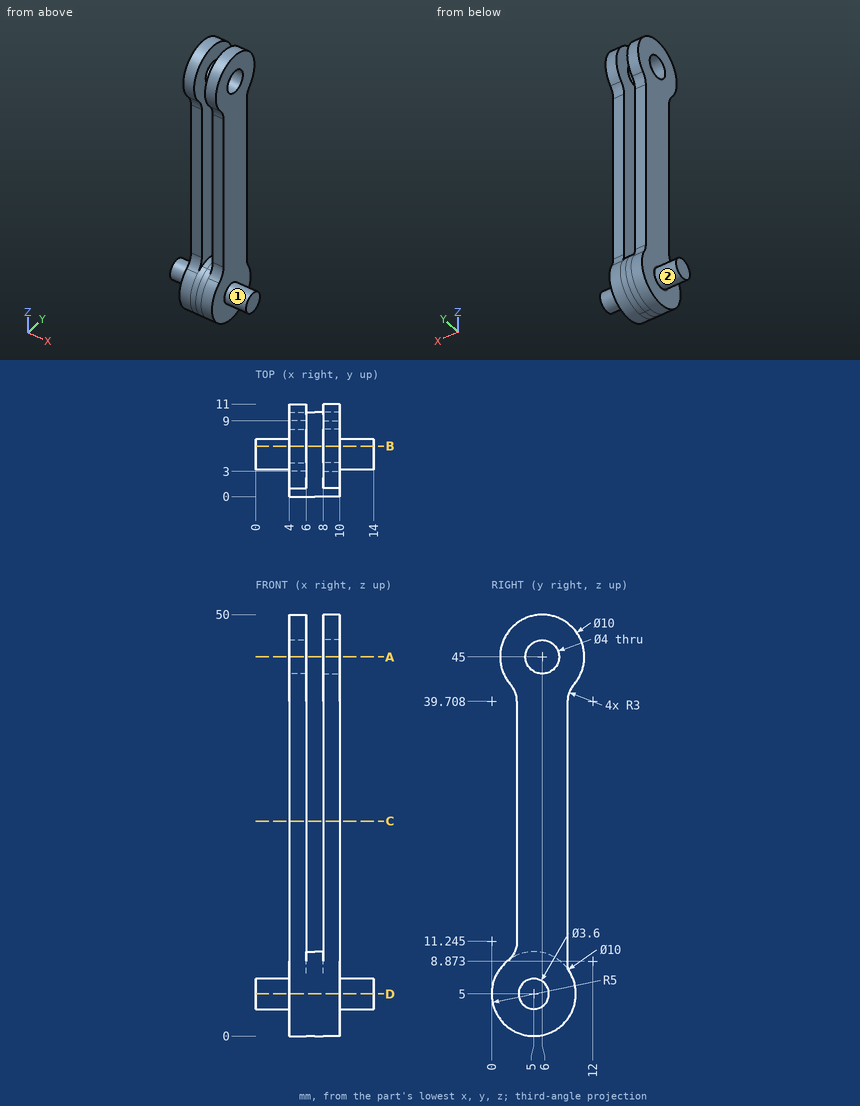
Design review of the part shown in the three views and the two pictorial views. Dimensions are in mm from the part's minimum x, y and z. A direction names the side the tool comes from. Give positions to 0.01 mm unless a question says otherwise; leave off trailing zeros. Loops run counter-clockwise (first coordinate to the right, second up) from the corner with the lowest first, then second, coordinate; pieces in that order, holes last. Notation, with made-up numbers: M 27,37.25 L 71,37.25 A26 cw 71,68.25 Z; hole C 76.5,79.5 d10. An arc over 180 degrees is marked long. Answer as a JSON object with one key per item and string values.
Item 1: We need section B-B (y = 6). State the section outline as (x, z) points.
Output values:
{"outline": "M 0,3.5 L 4,3.5 L 4,0.1 L 10,0.1 L 10,3.5 L 14,3.5 L 14,6.5 L 10,6.5 L 10,43 L 8,43 L 8,9.9 L 6,9.9 L 6,43 L 4,43 L 4,6.5 L 0,6.5 Z; M 4,47 L 6,47 L 6,50 L 4,50 Z; M 8,47 L 10,47 L 10,50 L 8,50 Z"}
Item 2: Machinability: for the marked faces 1 and 2, which of the approach directions +Z, -Z, +X, -X, +Y, -Y give a long, thin tool a straight path to every point of the face, cutting with its end or side? Answer none if there is none.
Output values:
{"face 1": "+X", "face 2": "-X"}
Item 3: We need section D-D (z = 5). State the section outline as (x, y) points.
Output values:
{"outline": "M 0,3.2 L 4,3.2 L 4,0 L 10,0 L 10,3.2 L 14,3.2 L 14,6.8 L 10,6.8 L 10,10 L 4,10 L 4,6.8 L 0,6.8 Z"}
Item 4: Wall thickness on line 1 along Y through (x, z) = (8.8, 45); line 2 along X through (y, z) = (5.75, 38); line 3 along X through (y, z) = (7, 8.5): over which ranges is each line inside the solid? List them lowest first.
Output values:
{"line 1": "y = 1 to 4, 8 to 11", "line 2": "x = 4 to 6, 8 to 10", "line 3": "x = 4 to 10"}
Item 5: We need section C-C (z = 25.5). State the section outline as (x, y) points.
Output values:
{"outline": "M 4,3 L 6,3 L 6,9 L 4,9 Z; M 8,3 L 10,3 L 10,9 L 8,9 Z"}
Item 6: For P1, Ø5.5, axis at y = 6.5, z = 33.5, coming from the -X side; P2, Ø1.5, axis at y = 4, z = 22, coming from the +X side; P3, Ø1.6, axis at x = 4.5, z = 23, coming from the +Y side, all flat-tipped, find the tip position at first contact; note any pin that passes through.
Output values:
{"P1": "stops at x = 4", "P2": "stops at x = 10", "P3": "stops at y = 9"}
Item 7: We need section A-A (z = 45). State the section outline as (x, y) points.
Output values:
{"outline": "M 4,1 L 6,1 L 6,4 L 4,4 Z; M 4,8 L 6,8 L 6,11 L 4,11 Z; M 8,1 L 10,1 L 10,4 L 8,4 Z; M 8,8 L 10,8 L 10,11 L 8,11 Z"}
